Work out the finished part from the listing and answer in its coordinate system (mm). Round coordinates to 2 decimals unless told otherwise and drop trailing zeros. Loops run counter-clockwise (first coordinate to the right, second up) from the corner with the lowest first, then second, coordinate; pieces in that order, holes last.
```python
from build123d import *

# Parameters (mm, degrees)
F1_DEPTH = 7
F4_R     = 60


with BuildPart() as f1:
    # F0 (on Front) → F1 (new body)
    with BuildSketch(Plane.XZ):
        with BuildLine():
            Line((-280, 0), (0, 0))
            Line((0, 0), (0, 400))
            Line((0, 400), (-300, 400))
            Line((-300, 400), (-300, 240))
            ThreePointArc((-300, 240), (-285.27864045, 222.360679775), (-280, 200))
            ThreePointArc((-280, 200), (-285.27864045, 177.639320225), (-300, 160))
            Line((-300, 160), (-300, 40))
            ThreePointArc((-300, 40), (-285.27864045, 22.360679775), (-280, 0))
        make_face()
    extrude(amount=F1_DEPTH)

    # F2: F1 across plane


with BuildPart() as f1_1:
    add(f1.part)
    add(f1.part.mirror(Plane.YZ))

    # F3: F1 across plane


with BuildPart() as f1_2:
    add(f1_1.part)
    add(f1_1.part.mirror(Plane.XY))

    # F4
    f4_edges = [f1_2.edges().sort_by_distance(p)[0] for p in [
        (-300, -3.5, 400),
        (300, -3.5, 400),
        (300, -3.5, -400),
        (-300, -3.5, -400),
    ]]
    fillet(f4_edges, radius=F4_R)


solid = f1_2.part
```
1. Given pin 1 (3 mm diameter, centred on x = -113, z = 137.5, fed in from +Y), flat-ended and moving along its own axis, determine where the tip first touches the part or whether it passes through.
Answer key:
pin 1: stops at y = 0
2. Find section B-B (z = 173). Write down the section's boundary in (x, y), then the cut area to 3 significant figures.
Answer key:
outline: (-287.92, -7) - (287.92, -7) - (287.92, 0) - (-287.92, 0) - close
area: 4,030 mm2
3. Determine the mould class of faces 1 (the face through (-281.96, -3.55, -382.89)), 2 (the face through (-282.89, -3.55, 381.96)), 3 (the face through (-280.004, -3.451, -200.649)) for opening direction Z: +Z half, -Z half, draft (parallel to the pull), parting line (faces both ways), or undercut.
Answer key:
face 1: -Z half
face 2: +Z half
face 3: undercut
4. Consider probe 1 along X at (y, z) = (-0.25, -196); probe 2 along X at (y, z) = (-1, -17); probe 3 along Z at (x, y) = (-260.5, -3.5). Determine where each line is inside the solid, lowest interval first.
Answer key:
probe 1: x = -280.16 to 280.16
probe 2: x = -282.98 to 282.98
probe 3: z = -396.39 to 396.39
5. Find section A-A (y = -3). Write down the section's boundary in (x, z).
Answer key:
outline: (-300, -340) arc R60 ccw to (-240, -400) - (240, -400) arc R60 ccw to (300, -340) - (300, -240) arc R50 cw to (300, -160) - (300, -40) arc R50 cw to (300, 40) - (300, 160) arc R50 cw to (300, 240) - (300, 340) arc R60 ccw to (240, 400) - (-240, 400) arc R60 ccw to (-300, 340) - (-300, 240) arc R50 cw to (-300, 160) - (-300, 40) arc R50 cw to (-300, -40) - (-300, -160) arc R50 cw to (-300, -240) - close
